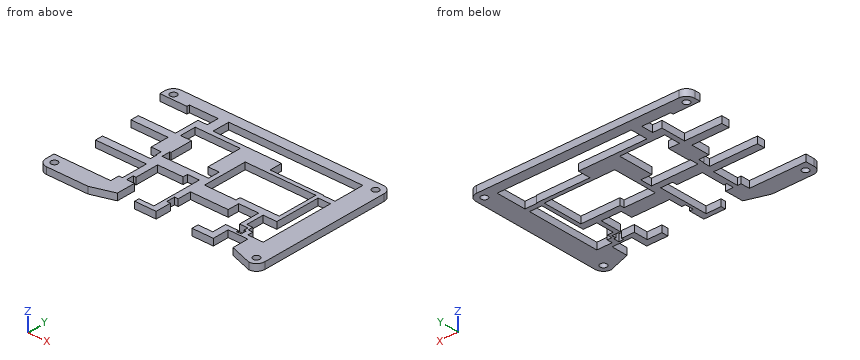
from build123d import *

# Parameters (mm, degrees)
BOSS_EXTRUDE1_OUTLINE_R = 1.3462
BOSS_EXTRUDE1_DEPTH     = 3.048
SKETCH14_W              = 2.2754
SKETCH14_H              = 2.1513
CUT_EXTRUDE2_DEPTH      = 430.898988368
SKETCH15_W              = 16.8402
SKETCH15_H              = 14.1197
SKETCH15_H_2            = 15.4101
CUT_EXTRUDE3_DEPTH      = 430.898988368
SKETCH16_R              = 1.524
CUT_EXTRUDE4_DEPTH      = 430.898988368


# Read off the part's stored shape, not the designer's step: Boss-Extrude1
with BuildPart() as part:
    # Boss-Extrude1 outline → Boss-Extrude1 (new body)
    with BuildSketch(Plane.XY):
        with BuildLine():
            ThreePointArc((-397.247125, 154.7804), (-399.946077222, 153.659592612), (-401.0571, 150.956597849))
            Line((-401.0571, 150.956597849), (-401.0571, 148.341))
            Line((-401.0571, 148.341), (-388.8032, 148.341))
            Line((-388.8032, 148.341), (-388.8032, 149.5347))
            Line((-388.8032, 149.5347), (-375.7222, 149.5347))
            Line((-375.7222, 149.5347), (-375.7222, 144.15))
            Line((-375.7222, 144.15), (-380.1672, 144.15))
            Line((-380.1672, 144.15), (-380.1672, 132.9309))
            Line((-380.1672, 132.9309), (-396.8172, 132.9309))
            Line((-396.8172, 132.9309), (-396.8172, 129.2706))
            Line((-396.8172, 129.2706), (-380.1672, 129.2706))
            Line((-380.1672, 129.2706), (-380.1672, 120.8224))
            Line((-380.1672, 120.8224), (-375.3812, 120.8224))
            Line((-375.3812, 120.8224), (-375.3812, 118.2824))
            Line((-375.3812, 118.2824), (-375.1272, 118.2824))
            Line((-375.1272, 118.2824), (-375.1272, 115.1509))
            Line((-375.1272, 115.1509), (-396.8172, 115.1509))
            Line((-396.8172, 115.1509), (-396.8172, 111.6447))
            Line((-396.8172, 111.6447), (-373.7775, 111.6447))
            Line((-373.7775, 111.6447), (-373.7775, 99.7089))
            Line((-373.7775, 99.7089), (-375.4172, 99.7089))
            Line((-375.4172, 99.7089), (-375.4172, 95.6449))
            Line((-375.4172, 95.6449), (-401.0571, 95.6449))
            Line((-401.0571, 95.6449), (-401.0571, 91.659304166))
            ThreePointArc((-401.0571, 91.659304166), (-399.951018769, 88.947400452), (-397.2472, 87.8217))
            Line((-397.2472, 87.8217), (-378.5565, 87.8217))
            Line((-378.5565, 87.8217), (-368.3165, 91.1883))
            Line((-368.3165, 91.1883), (-368.3165, 99.7089))
            Line((-368.3165, 99.7089), (-371.8725, 99.7089))
            Line((-371.8725, 99.7089), (-371.8725, 103.0109))
            Line((-371.8725, 103.0109), (-370.6025, 103.0109))
            Line((-370.6025, 103.0109), (-370.6025, 113.7612))
            Line((-370.6025, 113.7612), (-356.8152, 113.7612))
            Line((-356.8152, 113.7612), (-356.8152, 115.9125))
            Line((-356.8152, 115.9125), (-353.6872, 115.9125))
            Line((-353.6872, 115.9125), (-353.6872, 93.3059))
            Line((-353.6872, 93.3059), (-360.5003, 93.3059))
            Line((-360.5003, 93.3059), (-360.5003, 91.1883))
            Line((-360.5003, 91.1883), (-350.7686, 91.1883))
            Line((-350.7686, 91.1883), (-350.7686, 98.2843))
            Line((-350.7686, 98.2843), (-352.4372, 98.2843))
            Line((-352.4372, 98.2843), (-352.4372, 102.1451))
            Line((-352.4372, 102.1451), (-350.7686, 102.1451))
            Line((-350.7686, 102.1451), (-350.7686, 108.2665))
            Line((-350.7686, 108.2665), (-333.6613, 108.2665))
            Line((-333.6613, 108.2665), (-333.6613, 113.4801))
            Line((-333.6613, 113.4801), (-324.6295, 113.4801))
            Line((-324.6295, 113.4801), (-324.6295, 103.9551))
            Line((-324.6295, 103.9551), (-320.8233, 103.9551))
            Line((-320.8233, 103.9551), (-320.8233, 102.0978))
            Line((-320.8233, 102.0978), (-319.8913, 102.0978))
            Line((-319.8913, 102.0978), (-319.8913, 99.5578))
            Line((-319.8913, 99.5578), (-322.0933, 99.5578))
            Line((-322.0933, 99.5578), (-322.0933, 100.5738))
            Line((-322.0933, 100.5738), (-327.8337, 100.5738))
            Line((-327.8337, 100.5738), (-327.8337, 94.1717))
            Line((-327.8337, 94.1717), (-334.5393, 94.1717))
            Line((-334.5393, 94.1717), (-334.5393, 91.1883))
            Line((-334.5393, 91.1883), (-324.8873, 91.1883))
            Line((-324.8873, 91.1883), (-324.8873, 98.5911))
            Line((-324.8873, 98.5911), (-315.9973, 98.5911))
            Line((-315.9973, 98.5911), (-315.9973, 91.1883))
            Line((-315.9973, 91.1883), (-305.7573, 87.8217))
            ThreePointArc((-305.7573, 87.8217), (-303.063223164, 88.937623164), (-301.9473, 91.6317))
            Line((-301.9473, 91.6317), (-301.9473, 150.9704))
            ThreePointArc((-301.9473, 150.9704), (-303.063223164, 153.664476836), (-305.7573, 154.7804))
            Line((-305.7573, 154.7804), (-397.247125, 154.7804))
        make_face()
        with Locations((-397.2472, 91.6317)):
            Circle(BOSS_EXTRUDE1_OUTLINE_R, mode=Mode.SUBTRACT)
        with Locations((-305.7573, 91.6317)):
            Circle(BOSS_EXTRUDE1_OUTLINE_R, mode=Mode.SUBTRACT)
        Polygon((-322.5975, 105.3521), (-322.5975, 113.4801), (-316.4253, 113.4801), (-316.4253, 134.0739), (-310.8373, 134.0739), (-310.8373, 100.5738), (-317.7753, 100.5738), (-317.7753, 103.0869), (-319.8913, 103.0869), (-319.8913, 105.3521), align=None, mode=Mode.SUBTRACT)
        Polygon((-372.7142, 122.6512), (-372.7142, 132.9309), (-377.6672, 132.9309), (-377.6672, 140.2451), (-357.2832, 140.2451), (-357.2832, 124.1751), (-352.2032, 124.1751), (-352.2032, 118.8412), (-373.2222, 118.8412), (-373.2222, 122.6512), align=None, mode=Mode.SUBTRACT)
        with Locations((-397.247125, 150.9704)):
            Circle(BOSS_EXTRUDE1_OUTLINE_R, mode=Mode.SUBTRACT)
        Polygon((-335.9473, 116.6297), (-335.9473, 114.6425), (-350.1712, 114.6425), (-350.1712, 134.8668), (-318.2033, 134.8668), (-318.2033, 116.6297), align=None, mode=Mode.SUBTRACT)
        Polygon((-310.8374, 136.3599), (-316.4253, 136.3599), (-316.4253, 136.6448), (-340.5193, 136.6448), (-340.5193, 142.3597), (-371.5305, 142.3597), (-371.5305, 150.1697), (-310.8373, 150.1697), align=None, mode=Mode.SUBTRACT)
        with Locations((-305.7573, 150.9704)):
            Circle(BOSS_EXTRUDE1_OUTLINE_R, mode=Mode.SUBTRACT)
    extrude(amount=BOSS_EXTRUDE1_DEPTH)

    # Sketch14 → Cut-Extrude2 (cut, through all)
    with BuildSketch(Plane(origin=(0, 0, 0), x_dir=(-1, 0, 0), z_dir=(0, 0, -1))):
        with Locations((357.9529, 114.83685)):
            Rectangle(SKETCH14_W, SKETCH14_H)
    extrude(amount=-CUT_EXTRUDE2_DEPTH, mode=Mode.SUBTRACT)

    # Sketch15 → Cut-Extrude3 (cut, through all)
    with BuildSketch(Plane(origin=(0, 0, 0), x_dir=(-1, 0, 0), z_dir=(0, 0, -1))):
        with Locations((388.3971, 122.21075)):
            Rectangle(SKETCH15_W, SKETCH15_H)
        with Locations((388.3971, 140.63595)):
            Rectangle(SKETCH15_W, SKETCH15_H_2)
    extrude(amount=-CUT_EXTRUDE3_DEPTH, mode=Mode.SUBTRACT)

    # Sketch16 → Cut-Extrude4 (cut, through all)
    with BuildSketch(Plane.XY.offset(3.048)):
        with Locations((-397.247125, 150.9704)):
            Circle(SKETCH16_R)
        with Locations((-305.7573, 150.9704)):
            Circle(SKETCH16_R)
        with Locations((-305.7573, 91.6317)):
            Circle(SKETCH16_R)
        with Locations((-397.2472, 91.6317)):
            Circle(SKETCH16_R)
    extrude(amount=-CUT_EXTRUDE4_DEPTH, mode=Mode.SUBTRACT)


solid = part.part
Design review of the part built by this model. Coordinates are the model's own, in mm. Coordinates: 2 decimals unless noted, no trailing zeros. Loops run counter-clockwise (first coordinate to the right, second up) from the corner with the lowest first, then second, coordinate; pieces in that order, holes last. Notation, with made-up numbers: M 81,-32 L 114,-32 A20 cw 114,-28 Z; hole C 5.5,19.5 d4. An arc over 180 degrees is marked long. Answer as CSV lines item,"result".
Item 1: For P1, Ø1.5, axis at x = -337, z = 2, coming from the -Y side; P2, Ø10, axis at x = -382.5, y = 139, coming from the -Z side, all flat-tipped, find the tip position at first contact; note any pin that passes through.
Answer list:
P1,"y = 108.27"
P2,"z = 0"
Item 2: Add section A-A on x = -326. State the section outline as (y, z) points.
Answer list:
outline,"M 91.19,0 L 100.57,0 L 100.57,3.05 L 91.19,3.05 Z; M 113.48,0 L 116.63,0 L 116.63,3.05 L 113.48,3.05 Z; M 134.87,0 L 136.64,0 L 136.64,3.05 L 134.87,3.05 Z; M 150.17,0 L 154.78,0 L 154.78,3.05 L 150.17,3.05 Z"
Item 3: Add section B-B on x = -338. State the section outline as (y, z) points, plus the area to 3 significant figures.
Answer list:
outline,"M 108.27,0 L 114.64,0 L 114.64,3.05 L 108.27,3.05 Z; M 134.87,0 L 136.64,0 L 136.64,3.05 L 134.87,3.05 Z; M 150.17,0 L 154.78,0 L 154.78,3.05 L 150.17,3.05 Z"
area,"38.9 mm²"
Item 4: Add section C-C on y = 97. State the section outline as (x, z) points, plus the area to 3 significant figures.
Answer list:
outline,"M -375.42,0 L -368.32,0 L -368.32,3.05 L -375.42,3.05 Z; M -353.69,0 L -350.77,0 L -350.77,3.05 L -353.69,3.05 Z; M -327.83,0 L -324.89,0 L -324.89,3.05 L -327.83,3.05 Z; M -316,0 L -301.95,0 L -301.95,3.05 L -316,3.05 Z"
area,"82.3 mm²"
Item 5: For probe 1 along Y at (x, z) = (-392.5, 2); probe 2 along Y at (x, z) = (-338, 1.35); probe 3 along Y at (x, z) = (-325, 1.7), list the stretches that pass through material, from the lowest coordinate up.
Answer list:
probe 1,"87.82 to 95.64, 111.64 to 115.15, 129.27 to 132.93, 148.34 to 154.78"
probe 2,"108.27 to 114.64, 134.87 to 136.64, 150.17 to 154.78"
probe 3,"91.19 to 100.57, 113.48 to 116.63, 134.87 to 136.64, 150.17 to 154.78"
Item 6: Add section D-D on z = 1.75. Count the separate pieces of the cut face and the enclosed holes in it, plus the area to 3 significant figures.
Answer list:
separate pieces,"1"
enclosed holes,"8"
area,"2,440 mm²"
